```python
from build123d import *

# Parameters (mm, degrees)
F0_W     = 69.85
F0_H     = 44.45
F1_DEPTH = 4.7625
F2_R     = 3.175
F3_DEPTH = 25.4


with BuildPart() as f1:
    # F0 (on Front) → F1 (new body)
    with BuildSketch(Plane.XZ):
        Rectangle(F0_W, F0_H)
    extrude(amount=F1_DEPTH)

    # F2 (on face) → F3 (cut)
    with BuildSketch(Plane.XZ.offset(4.7625)):
        with BuildLine():
            ThreePointArc((-15.875, 3.175), (-19.05, 6.35), (-22.225, 3.175))
            ThreePointArc((-22.225, 3.175), (-19.05, 0), (-15.875, 3.175))
        make_face()
        with Locations((19.05, 3.175)):
            Circle(F2_R)
    extrude(amount=-F3_DEPTH, mode=Mode.SUBTRACT)


solid = f1.part
```
Could you check a few things on this model? Use its own coordinates, in mm. Give positions to 0.01 mm unless a question says otherwise; leave off trailing zeros. Loops run counter-clockwise (first coordinate to the right, second up) from the corner with the lowest first, then second, coordinate; pieces in that order, holes last. Notation, with made-up numbers: (17.5, 73.25) - (31.5, 73.25) arc R21 ccw to (31.5, 110.25) - close; hole circle Ø7 at (-30.75, -9). An arc over 180 degrees is marked (long way). Use one line per item in the form item = value.
1. I'm going to push a flat-ended pin straight in: pin 1 Ø4 at (x, z) = (-19.05, 3.175) entering from +Y. Where does the tip first touch, or does it pass through?
Response values:
pin_1 = through
2. I want a section at C-C (y = -3.55). Please give me the cut outline in (x, z) (3 decimals).
Response values:
outline = (-34.925, -22.225) - (34.925, -22.225) - (34.925, 22.225) - (-34.925, 22.225) - close; hole circle Ø6.35 at (-19.05, 3.175); hole circle Ø6.35 at (19.05, 3.175)
3. I want a section at B-B (z = 1). Please give me the cut outline in (x, y) (1 decimal), and give its area (3 significant figures).
Response values:
outline = (-34.9, -4.8) - (-21.4, -4.8) - (-21.4, 0) - (-34.9, 0) - close; (-16.7, -4.8) - (16.7, -4.8) - (16.7, 0) - (-16.7, 0) - close; (21.4, -4.8) - (34.9, -4.8) - (34.9, 0) - (21.4, 0) - close
area = 289 mm²
4. I need wall thicknesses on probe 1 along Z at (x, y) = (-19.05, -3.25) (3 decimals); probe 2 along X at (y, z) = (-1.75, 2.5) (3 decimals). Which ranges of each line are inside material? Lowest first, please.
Response values:
probe_1 = -22.225 to 0, 6.35 to 22.225
probe_2 = -34.925 to -22.152, -15.948 to 15.948, 22.152 to 34.925
5. Thinking about a two-plate mould opening in Z: for faces 1 (the face through (0, -2, -22.225)), 2 (the face through (-34.925, -2, 0)), 3 (the face through (15.878, -2.415, 3.315)), 4 (the face through (-15.878, -2.415, 3.035)), which applies, released by +Z, released by -Z, zero draft, split by the parting line, or undercut?
Response values:
face_1 = released by -Z
face_2 = zero draft
face_3 = undercut
face_4 = undercut
6. I want a section at D-D (x = -18.5). Please give me the cut outline in (y, z) (1 decimal).
Response values:
outline = (-4.8, -22.2) - (0, -22.2) - (0, 0) - (-4.8, 0) - close; (-4.8, 6.3) - (0, 6.3) - (0, 22.2) - (-4.8, 22.2) - close
